Verification items for the finished model (mm, model axes). Face numbers are marked on the shaded views. A direction names the side the tool comes from. Coordinates: 2 decimals unless noted, no trailing zeros. Loops run counter-clockwise (first coordinate to the right, second up) from the corner with the lowest first, then second, coordinate; pieces in that order, holes last. Notation, with made-up numbers: (69.5, 55) - (83.5, 55) arc R28 ccw to (83.5, 87) - close; hole circle Ø11 at (55.5, 51.25). An arc over 180 degrees is marked (long way). One line per item, written item: value. Start each with the question number.
(1) Section check A-A (x = 0). Record the boundary of the cut face in (y, z) (3 decimals).
(2) Section check D-D (y = 13). Record the boundary of the cut face in (x, z), plus the area to 3 significant figures.
(3) Section check C-C (y = 7.75). Record the boundary of the cut face in (x, z), plus the area to 3 significant figures.
(4) Set-up check for the marked faces 1, 2 and 3: record each of +Z, -Z, +X, -X, +Y, -Y from which the full face is reachable in a straight line by a thin tool's end or side.
(5) Thickness scan on probe 1 along Y at (x, z) = (-4, -1); probe 2 along Y at (x, z) = (2.5, -2.25); probe 3 along X at (y, z) = (3.75, 2). Record the ranges inside material, lowest first. Write a range as [from, to].
(6) Gauge pin test, flat ends, axial feed: P1, Ø1.5, axis at x = 0.5, y = 13.5, coming from the -Z side; P2, Ø5, axis at x = 1.5, y = 19.5, coming from the -Z side (3 decimals); P3, Ø2, axis at x = -2, y = 22.5, coming from the +Z side. Record the tip position at first contact, or that the pin passes through.
(7) Section check B-B (z = 0). Record the boundary of the cut face in (x, y) (3 decimals), plus the area to 3 significant figures.
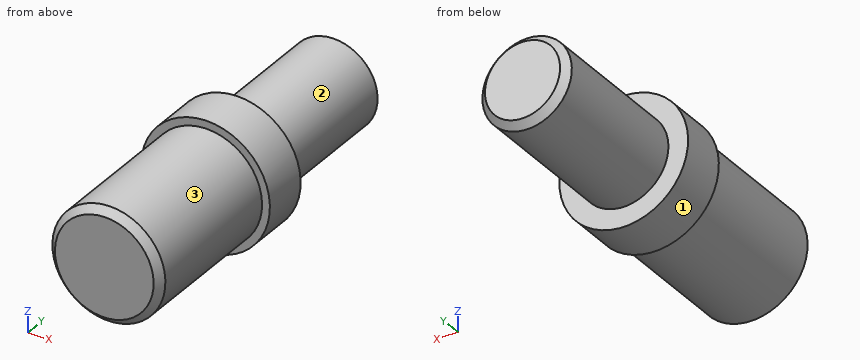
```python
from build123d import *

# Parameters (mm, degrees)
SKETCH1_R           = 3.95
BOSS_EXTRUDE1_DEPTH = 11
SKETCH2_R           = 4.5
BOSS_EXTRUDE2_DEPTH = 3.34
SKETCH4_R           = 3.125
BOSS_EXTRUDE3_DEPTH = 11
CHAMFER1_SIZE       = 0.5


with BuildPart() as part:
    # Sketch1 → Boss-Extrude1 (new body)
    with BuildSketch(Plane(origin=(0, 0, 0), x_dir=(1, 0, 0), z_dir=(0, 1, 0))):
        with Locations(Location((0, 0, 0), (0, 0, 270))):
            Circle(SKETCH1_R)
    extrude(amount=BOSS_EXTRUDE1_DEPTH)

    # Sketch2 → Boss-Extrude2 (add)
    with BuildSketch(Plane(origin=(0, 11, 0), x_dir=(1, 0, 0), z_dir=(0, 1, 0))):
        with Locations(Location((0, 0, 0), (0, 0, 270))):
            Circle(SKETCH2_R)
    extrude(amount=BOSS_EXTRUDE2_DEPTH)

    # Sketch4 → Boss-Extrude3 (add)
    with BuildSketch(Plane(origin=(0, 14.34, 0), x_dir=(1, 0, 0), z_dir=(0, 1, 0))):
        with Locations(Location((0, 0, 0), (0, 0, 270))):
            Circle(SKETCH4_R)
    extrude(amount=BOSS_EXTRUDE3_DEPTH)

    # Chamfer1
    chamfer1_edges = [part.edges().sort_by_distance(p)[0] for p in [
        (0, 25.34, -3.125),
        (0, 0, -3.95),
    ]]
    chamfer(chamfer1_edges, length=CHAMFER1_SIZE)


solid = part.part
```
Responses:
1. outline: (0, -3.45) - (0.5, -3.95) - (11, -3.95) - (11, -4.5) - (14.34, -4.5) - (14.34, -3.125) - (24.84, -3.125) - (25.34, -2.625) - (25.34, 2.625) - (24.84, 3.125) - (14.34, 3.125) - (14.34, 4.5) - (11, 4.5) - (11, 3.95) - (0.5, 3.95) - (0, 3.45) - close
2. outline: circle Ø9 at (0, 0)
2. area: 63.6 mm²
3. outline: circle Ø7.9 at (0, 0)
3. area: 49.0 mm²
4. face 1: +Y, -Y
4. face 2: +Y
4. face 3: -Y
5. probe 1: y = [11, 14.34]
5. probe 2: y = [0, 14.34]
5. probe 3: x = [-3.41, 3.41]
6. P1: stops at z = -4.5
6. P2: stops at z = -3.125
6. P3: stops at z = 2.96
7. outline: (-4.5, 11) - (-3.95, 11) - (-3.95, 0.5) - (-3.45, 0) - (3.45, 0) - (3.95, 0.5) - (3.95, 11) - (4.5, 11) - (4.5, 14.34) - (3.125, 14.34) - (3.125, 24.84) - (2.625, 25.34) - (-2.625, 25.34) - (-3.125, 24.84) - (-3.125, 14.34) - (-4.5, 14.34) - close
7. area: 185 mm²
